Input: part model. Units: mm. Frame: model coordinates. A direction names the side the tool comes from. Round coordinates to 2 decimals unless told otherwise and drop trailing zeros. Write each loop counter-clockwise with the first axis right and the second up, starting at its lowest first coordinate (ties: lowest second). Pieces come first, ordered by that corner, then holes. Notation, with made-up numbers: (75.5, -34) -> (86.5, -34) arc R30 ccw to (86.5, -3) -> close; hole circle Ø1 at (37.25, 65.25). An arc over 180 degrees is marked (long way). Write item = value, one per line.
Autodesk Inventor part; units mm, degrees
ref_plane "Work Plane2" through (-788.7937, -153, 28) normal (0, 0, 1) x (1, 0, 0)
ref_plane "YZ Plane" through (0, 0, 0) normal (1, 0, 0) x (0, 1, 0)
ref_plane "XZ Plane" through (0, 0, 0) normal (0, 1, 0) x (-1, 0, 0)
ref_plane "Work Plane1" through (0, 0, 0) normal (0, 0, 1) x (1, 0, 0)
sketch "Sketch1" plane through (0, 0, 0) normal (0, 0, 1) x (1, 0, 0)
  line L0 (-80.6325, -6) -> (-735.8557, -6)
  line L1 (-5.1227, -53.9222) -> (-80.6325, -6)
  line L2 (-1.3085, -54) -> (-4.8547, -54)
  line L3 (-58.1097, -2) -> (-0.9751, -53.1274)
  line L4 (-731.3557, -2) -> (-735.8557, -6)
  line L5 (-127.5657, -6) -> (-127.5657, 0)
  arc A0 (-5.1227, -53.9222) -> (-4.8547, -54) centre (-4.8547, -53.5) ccw
  arc A1 (-1.3085, -54) -> (-0.9751, -53.1274) centre (-1.3085, -53.5) ccw
  line L6 (-58.1097, -2) -> (-731.3557, -2)
  point P0 (0, 0)
  point P1 (-127.5657, -2)
ref_plane "Work Plane2" through (-788.7937, -153, 28) normal (0, 0, 1) x (1, 0, 0)
extrude "Extrusion1" add sketch "Sketch1" along normal up to surface (28 mm away) contours L0 L5 L6 L3 A1 L2 A0 L1
sketch "Sketch2" plane through (-127.5657, -6, 0) normal (0, -1, 0) x (1, 0, 0)
  circle A0 centre (27.1635, 14) radius 2.1
  line L0 (27.1635, 14) -> (30.6635, 14)
  line L1 (30.6635, 11.9793) -> (27.1635, 9.9585)
  line L2 (27.1635, 9.9585) -> (23.6635, 11.9793)
  line L3 (23.6635, 11.9793) -> (23.6635, 16.0207)
  line L4 (23.6635, 16.0207) -> (27.1635, 18.0415)
  line L5 (27.1635, 18.0415) -> (30.6635, 16.0207)
  line L6 (30.6635, 16.0207) -> (30.6635, 11.9793)
  point P0 (127.5657, 0)
  dimension "d2" = 3.5
extrude "Extrusion2" cut sketch "Sketch2" against normal blind 3.6 contours A0 | L6 L1 L2 L3 L4 L5
sketch "Sketch3" plane through (-127.5657, -2.4, 0) normal (0, -1, 0) x (1, 0, 0)
  line L0 (27.1635, 18.0415) -> (30.6635, 16.0207)
  line L1 (23.6635, 16.0207) -> (27.1635, 18.0415)
  line L2 (23.6635, 11.9793) -> (23.6635, 16.0207)
  line L3 (27.1635, 9.9585) -> (23.6635, 11.9793)
  line L4 (30.6635, 11.9793) -> (27.1635, 9.9585)
  line L5 (30.6635, 16.0207) -> (30.6635, 11.9793)
  circle A0 centre (27.1635, 14) radius 2.1
  point P0 (127.5657, 0)
  dimension "d5" = 4.2
extrude "Extrusion3" cut sketch "Sketch3" against normal through all contours A0
sketch "Sketch4" plane through (-127.5657, -6, 0) normal (0, -1, 0) x (1, 0, 0)
  line L0 (23.6635, 16.0207) -> (27.1635, 18.0415)
  line L1 (27.1635, 18.0415) -> (30.6635, 16.0207)
  line L2 (30.6635, 16.0207) -> (30.6635, 11.9793)
  line L3 (30.6635, 11.9793) -> (27.1635, 9.9585)
  line L4 (27.1635, 9.9585) -> (23.6635, 11.9793)
  line L5 (23.6635, 11.9793) -> (23.6635, 16.0207)
  line L6 (46.9332, 28) -> (0, 28)
  line L7 (0, 0) -> (0, 28)
  line L8 (0, 0) -> (46.9332, 0)
  line L9 (46.9332, 0) -> (46.9332, 28)
  line L10 (49.6735, 14) -> (46.1735, 14)
  line L11 (46.1735, 16.0207) -> (49.6735, 18.0415)
  line L12 (49.6735, 18.0415) -> (53.1735, 16.0207)
  line L13 (53.1735, 16.0207) -> (53.1735, 11.9793)
  line L14 (53.1735, 11.9793) -> (49.6735, 9.9585)
  line L15 (49.6735, 9.9585) -> (46.1735, 11.9793)
  line L16 (46.1735, 11.9793) -> (46.1735, 16.0207)
  circle A0 centre (49.6735, 14) radius 2.1
  line L17 (47.5735, 20) -> (47.5735, 10)
  arc A1 (47.5735, 10) -> (51.7735, 10) centre (49.6735, 10) ccw
  line L18 (51.7735, 10) -> (51.7735, 20)
  arc A2 (51.7735, 20) -> (47.5735, 20) centre (49.6735, 20) ccw
  line L19 (45.6735, 10) -> (45.6735, 20)
  arc A3 (53.6735, 20) -> (45.6735, 20) centre (49.6735, 20) ccw
  line L20 (53.6735, 10) -> (53.6735, 20)
  arc A4 (45.6735, 10) -> (53.6735, 10) centre (49.6735, 10) ccw
  point P0 (127.5657, 0)
  dimension "d8" = 3.5
  dimension "d9" = 4.2
extrude "Extrusion4" cut sketch "Sketch4" against normal up to surface (3.6 mm away) contours L11 L17 L10 L9 | L9 L10 L16 L11 | L10 L17 L15 L9 | L9 L15 L16 L10 | L11 L12 L18 A0 L17 | A0 | A0 L18 L14 L15 L17 | L18 L12 L13 L14
sketch "Sketch5" plane through (-127.5657, -6, 0) normal (0, -1, 0) x (1, 0, 0)
  line L0 (46.9332, 11.5407) -> (46.1735, 11.9793)
  line L1 (46.1735, 11.9793) -> (46.1735, 16.0207)
  line L2 (46.1735, 16.0207) -> (46.9332, 16.4593)
  line L3 (46.9332, 16.4593) -> (46.9332, 28)
  line L4 (46.9332, 28) -> (0, 28)
  line L5 (0, 0) -> (0, 28)
  line L6 (0, 0) -> (46.9332, 0)
  line L7 (46.9332, 0) -> (46.9332, 11.5407)
  line L8 (23.6635, 16.0207) -> (27.1635, 18.0415)
  line L9 (27.1635, 18.0415) -> (30.6635, 16.0207)
  line L10 (30.6635, 16.0207) -> (30.6635, 11.9793)
  line L11 (30.6635, 11.9793) -> (27.1635, 9.9585)
  line L12 (27.1635, 9.9585) -> (23.6635, 11.9793)
  line L13 (23.6635, 11.9793) -> (23.6635, 16.0207)
  line L14 (53.1735, 11.9793) -> (53.1735, 16.0207)
  line L15 (49.6735, 9.9585) -> (53.1735, 11.9793)
  circle A0 centre (49.6735, 14) radius 2.1
  point P0 (127.5657, 0)
extrude "Extrusion5" cut sketch "Sketch5" along normal blind 10 contours A0
sketch "Sketch6" plane through (-74.3922, -2.4, 11.9793) normal (0, -1, 0) x (1, 0, 0)
  line L0 (-7, 0) -> (-3.5, -2.0207)
  line L1 (-3.5, -2.0207) -> (0, 0)
  line L2 (0, 0) -> (0, 4.0415)
  line L3 (0, 4.0415) -> (-3.5, 6.0622)
  line L4 (-3.5, 6.0622) -> (-7, 4.0415)
  line L5 (-7, 4.0415) -> (-7, 0)
  point P0 (74.3922, -11.9793)
extrude "Extrusion6" cut sketch "Sketch6" along normal blind 10
sketch "Sketch7" plane through (-74.3922, -2.4, 11.9793) normal (0, -1, 0) x (1, 0, 0)
  circle A0 centre (-3.5, 2.0207) radius 2.1
  arc A1 (-3.5, -1.9793) -> (-3.5, 6.0207) centre (-3.5, 2.0207) ccw
  line L0 (-26.01, -1.9793) -> (-3.5, -1.9793)
  line L1 (-671.6821, 16.0207) -> (3.99, 16.0207)
  line L2 (3.99, -58.9793) -> (3.99, 16.0207)
  line L3 (-671.6821, -58.9793) -> (3.99, -58.9793)
  line L4 (-671.6821, -58.9793) -> (-671.6821, 16.0207)
  arc A2 (-30.01, -1.9793) -> (-22.01, -1.9793) centre (-26.01, -1.9793) ccw
  line L5 (-22.01, -1.9793) -> (-22.01, 8.0207)
  arc A3 (-22.01, 8.0207) -> (-30.01, 8.0207) centre (-26.01, 8.0207) ccw
  line L6 (-30.01, 8.0207) -> (-30.01, -1.9793)
  arc A4 (-7.5, -1.9793) -> (0.5, -1.9793) centre (-3.5, -1.9793) ccw
  line L7 (0.5, -1.9793) -> (0.5, 8.0207)
  arc A5 (0.5, 8.0207) -> (-7.5, 8.0207) centre (-3.5, 8.0207) ccw
  line L8 (-7.5, 8.0207) -> (-7.5, -1.9793)
  point P0 (74.3922, -11.9793)
extrude "Extrusion7" cut sketch "Sketch7" against normal blind 10 contours A0
sketch "Sketch8" plane through (-127.5657, -6, 0) normal (0, -1, 0) x (1, 0, 0)
  line L0 (46.9332, 11.5407) -> (46.1735, 11.9793)
  line L1 (46.1735, 11.9793) -> (46.1735, 16.0207)
  line L2 (46.1735, 16.0207) -> (46.9332, 16.4593)
  line L3 (46.9332, 16.4593) -> (46.9332, 28)
  line L4 (46.9332, 28) -> (0, 28)
  line L5 (0, 0) -> (0, 28)
  line L6 (0, 0) -> (46.9332, 0)
  line L7 (46.9332, 0) -> (46.9332, 11.5407)
  line L8 (23.6635, 16.0207) -> (27.1635, 18.0415)
  line L9 (27.1635, 18.0415) -> (30.6635, 16.0207)
  line L10 (30.6635, 16.0207) -> (30.6635, 11.9793)
  line L11 (30.6635, 11.9793) -> (27.1635, 9.9585)
  line L12 (27.1635, 9.9585) -> (23.6635, 11.9793)
  line L13 (23.6635, 11.9793) -> (23.6635, 16.0207)
  circle A0 centre (49.6735, 14) radius 5.3947
  line L14 (47.5735, 20) -> (47.5735, 10)
  arc A1 (47.5735, 10) -> (51.7735, 10) centre (49.6735, 10) ccw
  line L15 (51.7735, 10) -> (51.7735, 20)
  arc A2 (51.7735, 20) -> (47.5735, 20) centre (49.6735, 20) ccw
  line L16 (45.6735, 10) -> (45.6735, 20)
  arc A3 (53.6735, 20) -> (45.6735, 20) centre (49.6735, 20) ccw
  line L17 (53.6735, 10) -> (53.6735, 20)
  arc A4 (45.6735, 10) -> (53.6735, 10) centre (49.6735, 10) ccw
  point P0 (127.5657, 0)
  point P1 (46.9332, 9.3532)
  point P2 (46.9332, 18.6468)
extrude "Extrusion8" cut sketch "Sketch8" along normal blind 10 contours L0 L1 L2 L3 A0 L14 A1 L7 | A1 L14 A0 L15 | A1 L15 A0 L17 | L17 A0
ref_plane "Work Plane3" through (0, -54, -47) normal (-1, 0, 0) x (0, 0, 1)
sketch "Sketch9" plane through (0, -54, -47) normal (-1, 0, 0) x (0, 0, 1)
  line L0 (0, 0.8726) -> (47, 0.8726)
  line L1 (0, 63) -> (0, 0.8726)
  line L2 (0, 63) -> (75, 63)
  line L3 (75, 52) -> (75, 63)
  line L4 (47, 52) -> (47, 0.8726)
  line L5 (75, 52) -> (75, 0.8726)
  line L6 (47, 0.8726) -> (75, 0.8726)
  line L7 (47, 0.8726) -> (47, 52)
  line L8 (47, 54) -> (75, 54)
  line L9 (47, 0.8726) -> (47.3, 0.8726)
  line L10 (47.3, 0.8726) -> (47.3, 54)
  line L11 (47.3, 54) -> (47, 54)
  line L12 (47, 54) -> (47, 0.8726)
  line L13 (47, 52) -> (75, 52)
  line L14 (47, 52) -> (75, 52)
  dimension "d20" = 0.3
extrude "Extrusion9" cut sketch "Sketch9" along normal up to surface (127.5657 mm away) contours L4 L13 L10 L6 | L12 L8 L10 L13
properties part number "zaślepka-1"
1) Line query: L1, parallel to Y at x = -92.5, z = 19.25; L2, parallel to Y at x = -58, z = 11.5; L3, parallel to X at y = -7.7, z = 14. Output: solid intervals per line, ascending. Write a range as from..to.
Solutions:
L1 = -6..-2
L2 = -20.36..-2.1
L3 = -72.5..-51.74
2) Cut plane D-D (y = -34.5). Return the cut outline in (x, z).
Solutions:
outline = (-35.73, 0.3) -> (-21.79, 0.3) -> (-21.79, 28) -> (-35.73, 28) -> close
3) First-contact query: P1, Ø1, axis at y = -21.5, z = 8, coming from the -X side; P2, Ø10, axis at x = -14, z = 16.5, coming from the +Y side; P3, Ø8, axis at x = -54, z = 11, coming from the -Y side. Flat tips, straight axial feed; report the tip coordinate or a pass-through.
Solutions:
P1 = -57
P2 = -37
P3 = -25.44
4) Draft query along X for faces 1 (the face through (-79.618, -4.225, 10.955)), 2 (the face through (-42.349, -30.297, 13.804)), 3 (the face through (-79.618, -4.175, 17.045)), 4 (the face through (-92, -2, 14)). Return one class per face: +X half, -X half, draft (parallel to the pull), parting line (faces both ways), or undercut.
Solutions:
face_1 = undercut
face_2 = -X half
face_3 = undercut
face_4 = draft
5) Cut plane B-B (z = 24.25). Return the cut outline in (x, y), and give its area (3 significant figures).
Solutions:
outline = (-127.57, -6) -> (-80.63, -6) -> (-5.12, -53.92) arc R0.5 ccw to (-4.85, -54) -> (-1.31, -54) arc R0.5 ccw to (-0.98, -53.13) -> (-58.11, -2) -> (-127.57, -2) -> close
area = 1,050 mm^2
6) Access query for faces 5 (the face through (-102.128, -4.225, 10.955)), 6 (the face through (-55, -18, 28)). Directions: +Z, -Z, +X, -X, +Y, -Y. A direction counts if a zero-diameter tool reaches every point of the face in a straight line with its end or side. Return the directions, or none.
Solutions:
face_5 = -Y
face_6 = +Z, +X, -X, +Y, -Y
7) Cut plane C-C (x = -32.5). Return the cut outline in (y, z).
Solutions:
outline = (-36.55, 0.3) -> (-24.92, 0.3) -> (-24.92, 28) -> (-36.55, 28) -> close
8) Cut plane A-A (z = 14). Return the cut outline in (x, y), and give its area (3 significant figures).
Solutions:
outline = (-127.57, -6) -> (-103.9, -6) -> (-103.9, -2.4) -> (-102.5, -2.4) -> (-102.5, -2) -> (-127.57, -2) -> close; (-98.3, -2.4) -> (-96.9, -2.4) -> (-96.9, -6) -> (-81.39, -6) -> (-81.39, -2.4) -> (-79.99, -2.4) -> (-79.99, -2) -> (-98.3, -2) -> close; (-75.79, -2.4) -> (-74.39, -2.4) -> (-74.39, -6) -> (-72.5, -6) -> (-72.5, -11.16) -> (-5.12, -53.92) arc R0.5 ccw to (-4.85, -54) -> (-1.31, -54) arc R0.5 ccw to (-0.98, -53.13) -> (-58.11, -2) -> (-75.79, -2) -> close
area = 979 mm^2
